from build123d import *

# Parameters (mm, degrees)
PAD_DEPTH       = 2
SKETCH001_W     = 41.6
SKETCH001_H     = 41.6
PAD001_DEPTH    = 2
SKETCH002_W     = 2.3
SKETCH002_H     = 7
PAD002_DEPTH    = 7
SKETCH003_R     = 1.5
POCKET_DEPTH    = 45.820651
POCKET001_DEPTH = 2.001


with BuildPart() as part:
    # Sketch → Pad (new body)
    with BuildSketch(Plane.XY):
        with BuildLine():
            Line((-23.5, 21.719807), (-23.5, -21.719807))
            ThreePointArc((-23.5, -21.719807), (-22.627417, -22.627417), (-21.719807, -23.5))
            Line((-21.719807, -23.5), (21.719807, -23.5))
            ThreePointArc((21.719807, -23.5), (22.637656, -22.617174), (23.519651, -21.698526))
            Line((23.5, 21.719807), (23.519651, -21.698526))
            ThreePointArc((23.5, 21.719807), (22.627417, 22.627417), (21.719807, 23.5))
            Line((-21.719807, 23.5), (21.719807, 23.5))
            ThreePointArc((-21.719807, 23.5), (-22.627417, 22.627417), (-23.5, 21.719807))
        make_face()
    extrude(amount=PAD_DEPTH)

    # Sketch001 (on Face10 of Pad) → Pad001 (join)
    with BuildSketch(Plane.XY.offset(2)):
        with BuildLine():
            Line((-22.3, 21.244999), (-22.3, -21.244999))
            ThreePointArc((-22.3, -21.244999), (-21.778889, -21.778889), (-21.244999, -22.3))
            Line((-21.244999, -22.3), (21.244999, -22.3))
            ThreePointArc((21.244999, -22.3), (21.778889, -21.778889), (22.3, -21.244999))
            Line((22.3, 21.244999), (22.3, -21.244999))
            ThreePointArc((22.3, 21.244999), (21.778889, 21.778889), (21.244999, 22.3))
            Line((-21.244999, 22.3), (21.244999, 22.3))
            ThreePointArc((-21.244999, 22.3), (-21.778889, 21.778889), (-22.3, 21.244999))
        make_face()
        Rectangle(SKETCH001_W, SKETCH001_H, mode=Mode.SUBTRACT)
    extrude(amount=PAD001_DEPTH)

    # Sketch002 (on Face24 of Pad001) → Pad002 (join)
    with BuildSketch(Plane.XY.offset(2)):
        with Locations((-21.15, 0)):
            Rectangle(SKETCH002_W, SKETCH002_H)
        with Locations((21.15, 0)):
            Rectangle(SKETCH002_W, SKETCH002_H)
    extrude(amount=PAD002_DEPTH)

    # Sketch003 (on Face24 of Pad002) → Pocket (cut, through all)
    with BuildSketch(Plane(origin=(-22.3, 0, 0), x_dir=(0, -1, 0), z_dir=(-1, 0, 0))):
        with Locations((0, 6)):
            Circle(SKETCH003_R)
    extrude(amount=-POCKET_DEPTH, mode=Mode.SUBTRACT)

    # Sketch004 (on Face41 of Pocket) → Pocket001 (cut, through all)
    with BuildSketch(Plane.XY.offset(2)):
        with BuildLine():
            Line((-1.25, 18), (-1.25, -18))
            ThreePointArc((-5.25, -18), (-3.25, -20), (-1.25, -18))
            Line((-5.25, 18), (-5.25, -18))
            ThreePointArc((-1.25, 18), (-3.25, 20), (-5.25, 18))
        make_face()
        with BuildLine():
            Line((-7.75, 18), (-7.75, -18))
            ThreePointArc((-11.75, -18), (-9.75, -20), (-7.75, -18))
            Line((-11.75, 18), (-11.75, -18))
            ThreePointArc((-7.75, 18), (-9.75, 20), (-11.75, 18))
        make_face()
        with BuildLine():
            Line((-14.25, 18), (-14.25, -18))
            ThreePointArc((-18.25, -18), (-16.25, -20), (-14.25, -18))
            Line((-18.25, 18), (-18.25, -18))
            ThreePointArc((-14.25, 18), (-16.25, 20), (-18.25, 18))
        make_face()
        with BuildLine():
            Line((1.25, 18), (1.25, -18))
            ThreePointArc((1.25, -18), (3.25, -20), (5.25, -18))
            Line((5.25, 18), (5.25, -18))
            ThreePointArc((5.25, 18), (3.25, 20), (1.25, 18))
        make_face()
        with BuildLine():
            Line((7.75, 18), (7.75, -18))
            ThreePointArc((7.75, -18), (9.75, -20), (11.75, -18))
            Line((11.75, 18), (11.75, -18))
            ThreePointArc((11.75, 18), (9.75, 20), (7.75, 18))
        make_face()
        with BuildLine():
            Line((14.25, 18), (14.25, -18))
            ThreePointArc((14.25, -18), (16.25, -20), (18.25, -18))
            Line((18.25, 18), (18.25, -18))
            ThreePointArc((18.25, 18), (16.25, 20), (14.25, 18))
        make_face()
    extrude(amount=-POCKET001_DEPTH, mode=Mode.SUBTRACT)


solid = part.part
Design review of the part built by this model. Coordinates are the model's own, in mm. A direction names the side the tool comes from. Round coordinates to 2 decimals unless told otherwise and drop trailing zeros. Write each loop counter-clockwise with the first axis right and the second up, starting at its lowest first coordinate (ties: lowest second). Pieces come first, ordered by that corner, then holes. Notation, with made-up numbers: M 24,76 L 36,76 A17 cw 36,93 Z; hole C -10,62 d7. An arc over 180 degrees is marked long. One line per item, written item: value. Start each with the question number.
1. Clearance check with flat-ended pins moving along their axes: P1, Ø12, axis at x = 8.5, y = 16, coming from the -Z side; P2, Ø4, axis at x = 13.5, y = -5.5, coming from the +Z side; P3, Ø5, axis at x = 3, z = 6, coming from the +Y side; P4, Ø5, axis at y = -0.5, z = 1, coming from the +X side. State where each tip first meets the part, or that it passes through.
2. Draft analysis for pull direction X (two halves, no side actions). For faces 1 (the face through (-14.25, 0, 1)), 2 (the face through (-21.79, -21.77, 2.99)), 3 (the face through (20.8, -12, 3)), 4 (the face through (0, 23.5, 1)), state which applies: pulls with the +X half, pulls with the -X half, needs draft (parallel to the pull), parting line crosses it, or undercut.
3. Take a section at B-B on x = -3.25. State the section outline as (y, z) points.
4. For faces 5 (the face through (-21.166, 0.325, 4.536)), 6 (the face through (5.25, 0, 1)), 7 (the face through (0, 20.8, 3)), 8 (the face through (0, -21, 4)), list the 3-axis set-ups (+Z, -Z, +X, -X, +Y, -Y) from which the entire face can be reached by the end or side of a thin tool; tool diameter is ignored.
5. Take a section at A-A on z = 6. State the section outline as (x, y) points.
6. To check wall thickness, follow probe 1 along Y at (x, z) = (20.5, 2.5); probe 2 along X at (y, z) = (7, 3.5); probe 3 along Z at (x, y) = (-21.4, 0). State the ranges of each line that lie inside material, in increasing order. Write a range as from..to.
7. Take a section at C-C on x = 6.5. State the section outline as (y, z) points, then the cut area to 3 significant figures.
8. Take a section at D-D on y = 0. State how many separate pieces and enclosed holes the cut face has, then the cut area to 3 significant figures.
Computed:
1. P1: stops at z = 0
1. P2: stops at z = 2
1. P3: stops at y = 22.3
1. P4: stops at x = 23.51
2. face 1: undercut
2. face 2: pulls with the -X half
2. face 3: undercut
2. face 4: needs draft
3. outline: M -23.5,0 L -20,0 L -20,2 L -20.8,2 L -20.8,4 L -22.3,4 L -22.3,2 L -23.5,2 Z; M 20,0 L 23.5,0 L 23.5,2 L 22.3,2 L 22.3,4 L 20.8,4 L 20.8,2 L 20,2 Z
4. face 5: +X, -X
4. face 6: +Z, -Z
4. face 7: +Z
4. face 8: +Z, +X, -X, -Y
5. outline: M -22.3,-3.5 L -20,-3.5 L -20,-1.5 L -22.3,-1.5 Z; M -22.3,1.5 L -20,1.5 L -20,3.5 L -22.3,3.5 Z; M 20,-3.5 L 22.3,-3.5 L 22.3,-1.5 L 20,-1.5 Z; M 20,1.5 L 22.3,1.5 L 22.3,3.5 L 20,3.5 Z
6. probe 1: y = -22.3..-20.8, -3.5..3.5, 20.8..22.3
6. probe 2: x = -22.3..-20.8, 20.8..22.3
6. probe 3: z = 0..4.5, 7.5..9
7. outline: M -23.5,0 L 23.5,0 L 23.5,2 L 22.3,2 L 22.3,4 L 20.8,4 L 20.8,2 L -20.8,2 L -20.8,4 L -22.3,4 L -22.3,2 L -23.5,2 Z
7. area: 100 mm²
8. separate pieces: 9
8. enclosed holes: 0
8. area: 64.4 mm²
